Part print with two shaded views. Sizes in mm from the minimum x, y, z corner. A direction names the side the tool comes from. Round coordinates to 2 decimals unless told otherwise and drop trailing zeros. Order: outer loops, then holes, each group sorted by start corner. A loop starts at its lowest first (then second) coordinate and runs counter-clockwise, first axis right, second up. Notation, with made-up numbers: (47, 66) - (79, 66) arc R34 ccw to (79, 98) - close; hole circle Ø5 at (23, 88.5). An arc over 180 degrees is marked (long way). Write item = value, one per line.
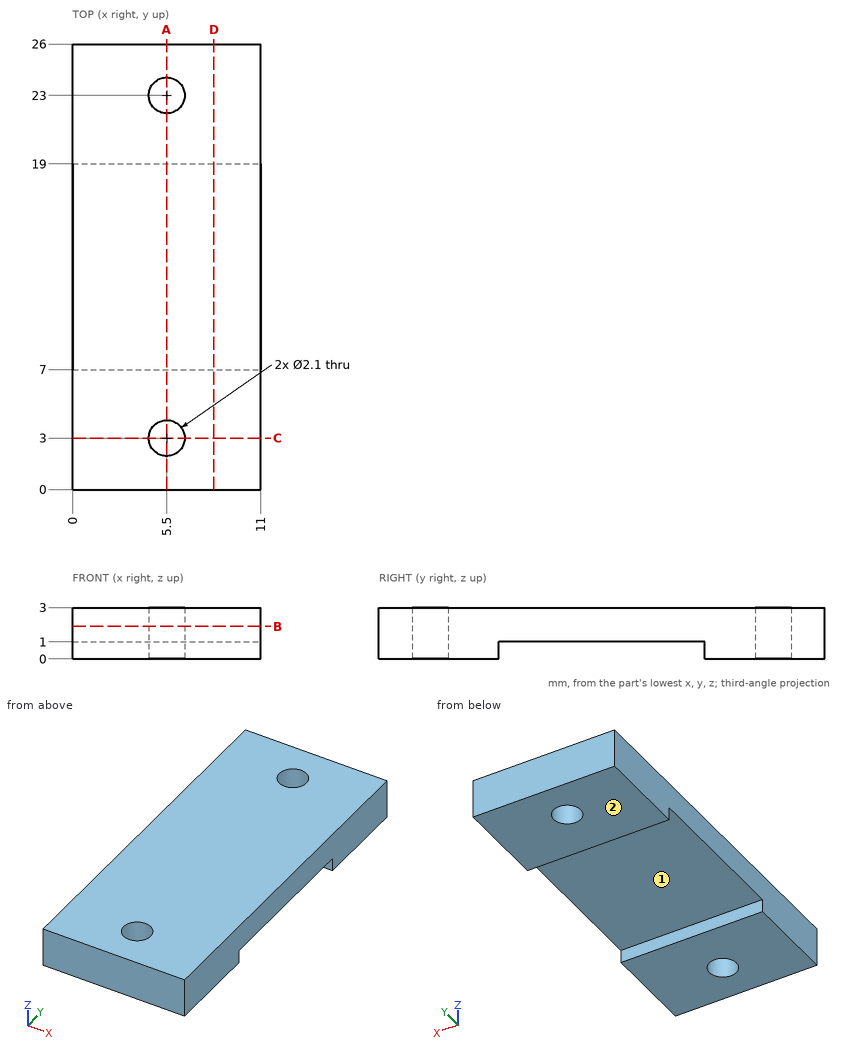
1) Cut at D-D (x = 8.25). Write the cut outline in (y, z), and give its area (3 significant figures).
Conclusion:
outline = (0, 0) - (7, 0) - (7, 1) - (19, 1) - (19, 0) - (26, 0) - (26, 3) - (0, 3) - close
area = 66.0 mm^2
2) 3-axis set-ups, long thin cutter, end or side, ignore diameter. For the marked faces 1 and 2: which of +Z, -Z, +X, -X, +Y, -Y reach the whole face in a straight line?
Conclusion:
face_1 = -Z, +X, -X
face_2 = -Z, +X, -X, +Y, -Y
3) Cut at B-B (z = 1.9). Write the cut outline in (x, y), and give its area (3 significant figures).
Conclusion:
outline = (0, 0) - (11, 0) - (11, 26) - (0, 26) - close; hole circle Ø2.1 at (5.5, 3); hole circle Ø2.1 at (5.5, 23)
area = 279 mm^2
4) Cut at C-C (y = 3). Write the cut outline in (x, z).
Conclusion:
outline = (0, 0) - (4.45, 0) - (4.45, 3) - (0, 3) - close; (6.55, 0) - (11, 0) - (11, 3) - (6.55, 3) - close
5) Cut at A-A (x = 5.5). Write the cut outline in (y, z).
Conclusion:
outline = (0, 0) - (1.95, 0) - (1.95, 3) - (0, 3) - close; (4.05, 0) - (7, 0) - (7, 1) - (19, 1) - (19, 0) - (21.95, 0) - (21.95, 3) - (4.05, 3) - close; (24.05, 0) - (26, 0) - (26, 3) - (24.05, 3) - close
6) Wall check: line 1 along Y through (x, z) = (5.5, 0.65); line 2 along Y through (x, z) = (1, 0.45); line 3 along Z through (x, y) = (9, 12.75). Give the ranges that are in metal, low to high.
Conclusion:
line_1 = 0 to 1.95, 4.05 to 7, 19 to 21.95, 24.05 to 26
line_2 = 0 to 7, 19 to 26
line_3 = 1 to 3
